```python
from build123d import *

# Parameters (mm, degrees)
F0_W     = 50
F0_H     = 700
F1_DEPTH = 50
F2_F1_R  = 2
F2_F2_R  = 2
F2_F3_R  = 2


with BuildPart() as f1:
    # F0 (on Front) → F1 (new body)
    with BuildSketch(Plane.XZ):
        Polygon((1200, 0), (0, 0), (0, -50), (50, -50), (1150, -50), (1200, -50), align=None)
        with Locations((25, -400)):
            Rectangle(F0_W, F0_H)
        Polygon((50, -750), (0, -750), (0, -800), (1200, -800), (1200, -750), (1150, -750), align=None)
        with Locations((1175, -400)):
            Rectangle(F0_W, F0_H)
    extrude(amount=F1_DEPTH)

    # F2: fillet of radius 2 on 22 edges, made by hand

    # F2_f1
    f2_f1_edges = [f1.edges().sort_by_distance(p)[0] for p in [
        (50, -25, -50),
        (1150, -25, -50),
        (1150, -25, -750),
        (50, -25, -750),
    ]]
    fillet(f2_f1_edges, radius=F2_F1_R)

    # F2_f2
    f2_f2_edges = [f1.edges().sort_by_distance(p)[0] for p in [
        (600, -50, 0),
        (1200, -25, 0),
        (1200, -50, -400),
        (1200, 0, -400),
        (600, 0, 0),
        (0, 0, -400),
        (600, 0, -800),
        (600, -50, -50),
        (600, -50, -750),
        (0, -25, -800),
        (1200, -25, -800),
        (600, -50, -800),
        (0, -25, 0),
        (0, -50, -400),
        (1149.4142135624, -50, -749.4142135624),
        (50.5857864376, -50, -749.4142135624),
        (50.5857864376, -50, -50.5857864376),
        (1149.4142135624, -50, -50.5857864376),
    ]]
    fillet(f2_f2_edges, radius=F2_F2_R)

    # F2_f3
    f2_f3_edges = [f1.edges().sort_by_distance(p)[0] for p in [
        (600, 0, -750),
        (50, 0, -400),
        (600, 0, -50),
        (1150, 0, -400),
        (1149.4142135624, 0, -50.5857864376),
        (1149.4142135624, 0, -749.4142135624),
        (50.5857864376, 0, -50.5857864376),
        (50.5857864376, 0, -749.4142135624),
    ]]
    fillet(f2_f3_edges, radius=F2_F3_R)


solid = f1.part
```
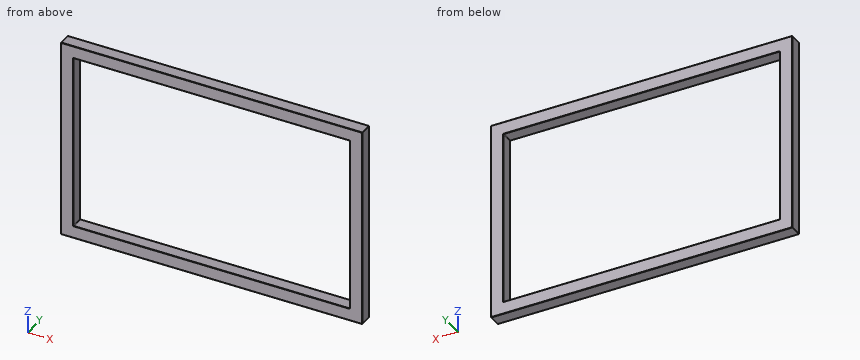
Input: part model. Units: mm. Frame: model coordinates. Give positions to 0.01 mm unless a question says otherwise; leave off trailing zeros. Loops run counter-clockwise (first coordinate to the right, second up) from the corner with the lowest first, then second, coordinate; pieces in that order, holes last.
1) Section query B-B on x = 1001. Return the cut outline in (y, z), and give its area (3 significant figures).
A:
outline: (-50, -798) arc R2 ccw to (-48, -800) - (-2, -800) arc R2 ccw to (0, -798) - (0, -752) arc R2 ccw to (-2, -750) - (-48, -750) arc R2 ccw to (-50, -752) - close; (-50, -48) arc R2 ccw to (-48, -50) - (-2, -50) arc R2 ccw to (0, -48) - (0, -2) arc R2 ccw to (-2, 0) - (-48, 0) arc R2 ccw to (-50, -2) - close
area: 4,990 mm2
2) Section query A-A on y = -18.5. Return the cut outline in (x, z), and give its area (3 significant figures).
A:
outline: (0, -798) arc R2 ccw to (2, -800) - (1198, -800) arc R2 ccw to (1200, -798) - (1200, -2) arc R2 ccw to (1198, 0) - (2, 0) arc R2 ccw to (0, -2) - close; hole (50, -748) arc R2 ccw to (52, -750) - (1148, -750) arc R2 ccw to (1150, -748) - (1150, -52) arc R2 ccw to (1148, -50) - (52, -50) arc R2 ccw to (50, -52) - close
area: 190,000 mm2
3) Line query: L1, parallel to X at y = -5.5, z = -662; L2, parallel to Z at x = 550, y = -41.5. Output: solid intervals per line, ascending.
A:
L1: x = 0 to 50, 1150 to 1200
L2: z = -800 to -750, -50 to 0
4) Section query C-C on z = -602.5. Return the cut outline in (x, y), and give its area (3 significant figures).
A:
outline: (0, -48) arc R2 ccw to (2, -50) - (48, -50) arc R2 ccw to (50, -48) - (50, -2) arc R2 ccw to (48, 0) - (2, 0) arc R2 ccw to (0, -2) - close; (1150, -48) arc R2 ccw to (1152, -50) - (1198, -50) arc R2 ccw to (1200, -48) - (1200, -2) arc R2 ccw to (1198, 0) - (1152, 0) arc R2 ccw to (1150, -2) - close
area: 4,990 mm2
